Read the model definition and answer for the solid it produces. Units are mm, in the model's axes. A direction names the side the tool comes from. Coordinates: 2 decimals unless noted, no trailing zeros. Write each loop counter-clockwise with the first axis right and the second up, starting at its lowest first coordinate (ties: lowest second). Pieces come first, ordered by that corner, then holes. Notation, with made-up numbers: (72.5, -33) -> (78.5, -33) arc R24 ccw to (78.5, -8) -> close; hole circle Ø10 at (20, 64). An arc over 180 degrees is marked (long way). Return JSON: item names as keys, results as strings.
from build123d import *

# Parameters (mm, degrees)
BOSS_EXTRUDE2_DEPTH      = 12.5
BOSS_EXTRUDE2_DEPTH_BACK = 12.5
SKETCH2_R                = 3.25
CUT_EXTRUDE3_DEPTH       = 45


with BuildPart() as part:
    # Sketch1 → Boss-Extrude2 (new, two sides: drawn at the far end of the back side and taken through both)
    with BuildSketch(Plane.XY.offset(-BOSS_EXTRUDE2_DEPTH_BACK)):
        with BuildLine():
            Line((87.5, 0), (-87.5, 0))
            Line((-87.5, 0), (-87.5, 5))
            Line((-87.5, 5), (-49.996574748, 5))
            ThreePointArc((-49.996574748, 5), (-45.686739788, 5.89034852), (-43.75, 9.842112287))
            Line((-43.75, 9.842112287), (-43.75, 45))
            Line((-43.75, 45), (-22.5, 45))
            Line((-22.5, 45), (-22.5, 35))
            Line((-22.5, 35), (-18.5, 35))
            ThreePointArc((-18.5, 35), (0, 16.5), (18.5, 35))
            Line((18.5, 35), (22.5, 35))
            Line((22.5, 35), (22.5, 45))
            Line((22.5, 45), (43.75, 45))
            Line((43.75, 45), (43.75, 9.842112287))
            ThreePointArc((43.75, 9.842112287), (45.686739788, 5.89034852), (49.996574748, 5))
            Line((49.996574748, 5), (87.5, 5))
            Line((87.5, 5), (87.5, 0))
        make_face()
    extrude(amount=BOSS_EXTRUDE2_DEPTH + BOSS_EXTRUDE2_DEPTH_BACK)

    # Sketch2 → Cut-Extrude3 (cut)
    with BuildSketch(Plane(origin=(0, 0, 0), x_dir=(1, 0, 0), z_dir=(0, 1, 0))):
        with Locations(Location((-30.5, 0, 0), (0, 0, 90))):
            Circle(SKETCH2_R)
        with Locations(Location((30.5, 0, 0), (0, 0, 90))):
            Circle(SKETCH2_R)
        with BuildLine():
            Line((-72.502650664, 5), (-62.502650664, 5))
            ThreePointArc((-62.502650664, 5), (-57.502650664, 0), (-62.502650664, -5))
            Line((-62.502650664, -5), (-72.502650664, -5))
            ThreePointArc((-72.502650664, -5), (-77.502650664, 0), (-72.502650664, 5))
        make_face()
        with BuildLine():
            Line((72.502650664, -5), (62.502650664, -5))
            ThreePointArc((62.502650664, -5), (57.502650664, 0), (62.502650664, 5))
            Line((62.502650664, 5), (72.502650664, 5))
            ThreePointArc((72.502650664, 5), (77.502650664, 0), (72.502650664, -5))
        make_face()
    extrude(amount=CUT_EXTRUDE3_DEPTH, mode=Mode.SUBTRACT)


solid = part.part
1. The part is cut by section C-C (x = 30.5). Determine the outline of the cut face in (y, z), then the cut area to 4 significant figures.
Taken from the geometry:
{"outline": "(0, -12.5) -> (45, -12.5) -> (45, -3.25) -> (0, -3.25) -> close; (0, 3.25) -> (45, 3.25) -> (45, 12.5) -> (0, 12.5) -> close", "area": "832.5 mm2"}
2. Consider L1, parallel to X at y = 12, z = 0; L2, parallel to X at y = 36.5, z = 0; L3, parallel to X at y = 37, z = 9.25. Determine where each line is inside the solid, lowest interval first.
Taken from the geometry:
{"L1": "x = -43.75 to -33.75, -27.25 to 27.25, 33.75 to 43.75", "L2": "x = -43.75 to -33.75, -27.25 to -22.5, 22.5 to 27.25, 33.75 to 43.75", "L3": "x = -43.75 to -22.5, 22.5 to 43.75"}
3. A tool of negligible diameter and unlimited length cuts with its end or side. For faces 1 (the face through (-57.504, 2.465, -0.11)), 2 (the face through (-22.5, 40, 0)), 3 (the face through (-43.75, 27, 0)), from which of +Z, -Z, +X, -X, +Y, -Y can it reach the whole face along a straight path? Write none if from no direction.
Taken from the geometry:
{"face 1": "+Y, -Y", "face 2": "+Z, -Z, +Y", "face 3": "+Z, -Z, -X, +Y"}
4. The part is cut by section A-A (y = 41). Determine the outline of the cut face in (x, z), then the cut area to 3 significant figures.
Taken from the geometry:
{"outline": "(-43.75, -12.5) -> (-22.5, -12.5) -> (-22.5, 12.5) -> (-43.75, 12.5) -> close; (22.5, -12.5) -> (43.75, -12.5) -> (43.75, 12.5) -> (22.5, 12.5) -> close; hole circle Ø6.5 at (-30.5, 0); hole circle Ø6.5 at (30.5, 0)", "area": "996 mm2"}
5. For a pull along Z with two mould halves and no side action, classify faces 4 (the face through (45.637, 5.93, -0.175)), 5 (the face through (67, 2, -5)) as +Z half, -Z half, draft (parallel to the pull), parting line (faces both ways), or undercut.
Taken from the geometry:
{"face 4": "draft", "face 5": "undercut"}
6. The part is cut by section B-B (z = 0). Count the separate pieces of the cut face and the enclosed holes in it, then the cut area to 3 significant figures.
Taken from the geometry:
{"separate pieces": "5", "enclosed holes": "0", "area": "2,610 mm2"}
7. The part is cut by section D-D (y = 11.5). Determine the outline of the cut face in (x, z), then the cut area to 3 significant figures.
Taken from the geometry:
{"outline": "(-43.75, -12.5) -> (43.75, -12.5) -> (43.75, 12.5) -> (-43.75, 12.5) -> close; hole circle Ø6.5 at (-30.5, 0); hole circle Ø6.5 at (30.5, 0)", "area": "2,120 mm2"}
8. Flat-ended cylindrical pins translate along their axes: pin 1 Ø8 at (y, z) = (42, -4) entering from +X; pin 2 Ø4 at (x, z) = (-1.5, -5.5) entering from +Y; pin 3 Ø1 at (x, y) = (-45, 32) entering from +Z; pin 4 Ø12.5 at (x, z) = (67.5, 3.5) entering from +Y. Find the tip coordinate at first contact, or state that the pin passes through.
Taken from the geometry:
{"pin 1": "stops at x = 43.75", "pin 2": "stops at y = 16.83", "pin 3": "passes through", "pin 4": "stops at y = 5"}
